```python
from build123d import *

# Parameters (mm, degrees)
SKETCH2_R               = 1.4
BOSS_EXTRUDE1_DEPTH     = 1.5
SKETCH5_R               = 1.6
CUT_EXTRUDE1_DEPTH      = 0.5
SKETCH3_R               = 1.4
SKETCH3_W               = 32.6
SKETCH3_H               = 52.5
BOSS_EXTRUDE2_DEPTH     = 1.5
SKETCH4_R               = 1.4
BOSS_EXTRUDE3_DEPTH     = 13.5
CHAMFER1_SIZE           = 2
CUT_EXTRUDE2_DEPTH      = 1
CUT_EXTRUDE2_DEPTH_BACK = 2.5


with BuildPart() as part:
    # Sketch2 → Boss-Extrude1 (new body)
    with BuildSketch(Plane(origin=(0, 0, 0), x_dir=(1, 0, 0), z_dir=(0, 1, 0))):
        with BuildLine():
            Line((-1.5, -1.5), (-1.5, 4.9))
            Line((-1.5, 4.9), (-4, 7.4))
            Line((-4, 7.4), (-4.5, 7.4))
            ThreePointArc((-4.5, 7.4), (-8.6, 11.5), (-4.5, 15.6))
            Line((-4.5, 15.6), (-4, 15.6))
            Line((-4, 15.6), (-1.5, 18.1))
            Line((-1.5, 18.1), (-1.5, 35.4))
            Line((-1.5, 35.4), (-4, 37.9))
            Line((-4, 37.9), (-4.5, 37.9))
            ThreePointArc((-4.5, 37.9), (-8.6, 42), (-4.5, 46.1))
            Line((-4.5, 46.1), (-4, 46.1))
            Line((-4, 46.1), (-1.5, 48.6))
            Line((-1.5, 48.6), (-1.5, 53.5))
            Line((-1.5, 53.5), (33.6, 53.5))
            Line((33.6, 53.5), (33.6, 48.6))
            Line((33.6, 48.6), (36.1, 46.1))
            Line((36.1, 46.1), (36.6, 46.1))
            ThreePointArc((36.6, 46.1), (40.7, 42), (36.6, 37.9))
            Line((36.6, 37.9), (36.1, 37.9))
            Line((36.1, 37.9), (33.6, 35.4))
            Line((33.6, 35.4), (33.6, 18.1))
            Line((33.6, 18.1), (36.1, 15.6))
            Line((36.1, 15.6), (36.6, 15.6))
            ThreePointArc((36.6, 15.6), (40.7, 11.5), (36.6, 7.4))
            Line((36.6, 7.4), (36.1, 7.4))
            Line((36.1, 7.4), (33.6, 4.9))
            Line((33.6, 4.9), (33.6, -1.5))
            Line((33.6, -1.5), (-1.5, -1.5))
        make_face()
        with Locations((-4.5, 42)):
            Circle(SKETCH2_R, mode=Mode.SUBTRACT)
        with Locations((-4.5, 11.5)):
            Circle(SKETCH2_R, mode=Mode.SUBTRACT)
        with Locations((36.6, 11.5)):
            Circle(SKETCH2_R, mode=Mode.SUBTRACT)
        with Locations((36.6, 42)):
            Circle(SKETCH2_R, mode=Mode.SUBTRACT)
    extrude(amount=-BOSS_EXTRUDE1_DEPTH)

    # Sketch5 → Cut-Extrude1 (cut)
    with BuildSketch(Plane(origin=(0, 0, 0), x_dir=(1, 0, 0), z_dir=(0, 1, 0))):
        with Locations((2.5, 42)):
            Circle(SKETCH5_R)
        with Locations((29.6, 42)):
            Circle(SKETCH5_R)
        with Locations((29.6, 11.5)):
            Circle(SKETCH5_R)
        with Locations((2.5, 11.5)):
            Circle(SKETCH5_R)
        Polygon((14.55, 36), (17.55, 36), (17.55, 39), (19.05, 39), (16.05, 42), (13.05, 39), (14.55, 39), align=None)
    extrude(amount=-CUT_EXTRUDE1_DEPTH, mode=Mode.SUBTRACT)

    # Sketch3 → Boss-Extrude2 (add)
    with BuildSketch(Plane(origin=(0, 0, 0), x_dir=(1, 0, 0), z_dir=(0, 1, 0))):
        with BuildLine():
            Line((-1.5, 53.5), (33.6, 53.5))
            Line((33.6, 53.5), (33.6, 48.6))
            Line((33.6, 48.6), (36.1, 46.1))
            Line((36.1, 46.1), (36.6, 46.1))
            ThreePointArc((36.6, 46.1), (40.7, 42), (36.6, 37.9))
            Line((36.6, 37.9), (36.1, 37.9))
            Line((36.1, 37.9), (33.6, 35.4))
            Line((33.6, 35.4), (33.6, 18.1))
            Line((33.6, 18.1), (36.1, 15.6))
            Line((36.1, 15.6), (36.6, 15.6))
            ThreePointArc((36.6, 15.6), (40.7, 11.5), (36.6, 7.4))
            Line((36.6, 7.4), (36.1, 7.4))
            Line((36.1, 7.4), (33.6, 4.9))
            Line((33.6, 4.9), (33.6, -1.5))
            Line((33.6, -1.5), (-1.5, -1.5))
            Line((-1.5, -1.5), (-1.5, 4.9))
            Line((-1.5, 4.9), (-4, 7.4))
            Line((-4, 7.4), (-4.5, 7.4))
            ThreePointArc((-4.5, 7.4), (-8.6, 11.5), (-4.5, 15.6))
            Line((-4.5, 15.6), (-4, 15.6))
            Line((-4, 15.6), (-1.5, 18.1))
            Line((-1.5, 18.1), (-1.5, 35.4))
            Line((-1.5, 35.4), (-4, 37.9))
            Line((-4, 37.9), (-4.5, 37.9))
            ThreePointArc((-4.5, 37.9), (-8.6, 42), (-4.5, 46.1))
            Line((-4.5, 46.1), (-4, 46.1))
            Line((-4, 46.1), (-1.5, 48.6))
            Line((-1.5, 48.6), (-1.5, 53.5))
        make_face()
        with Locations((-4.5, 42)):
            Circle(SKETCH3_R, mode=Mode.SUBTRACT)
        with Locations((36.6, 42)):
            Circle(SKETCH3_R, mode=Mode.SUBTRACT)
        with Locations((36.6, 11.5)):
            Circle(SKETCH3_R, mode=Mode.SUBTRACT)
        with Locations((-4.5, 11.5)):
            Circle(SKETCH3_R, mode=Mode.SUBTRACT)
        with Locations((16.05, 26)):
            Rectangle(SKETCH3_W, SKETCH3_H, mode=Mode.SUBTRACT)
    extrude(amount=BOSS_EXTRUDE2_DEPTH)

    # Sketch4 → Boss-Extrude3 (add)
    with BuildSketch(Plane(origin=(0, 1.5, 0), x_dir=(1, 0, 0), z_dir=(0, 1, 0))):
        with BuildLine():
            Line((-4.5, 46.1), (-0.25, 46.1))
            Line((-0.25, 46.1), (-0.25, 37.9))
            Line((-0.25, 37.9), (-4.5, 37.9))
            ThreePointArc((-4.5, 37.9), (-8.6, 42), (-4.5, 46.1))
        make_face()
        with Locations((-4.5, 42)):
            Circle(SKETCH4_R, mode=Mode.SUBTRACT)
        with BuildLine():
            Line((-4.5, 7.4), (-0.25, 7.4))
            Line((-0.25, 7.4), (-0.25, 15.6))
            Line((-0.25, 15.6), (-4.5, 15.6))
            ThreePointArc((-4.5, 15.6), (-8.6, 11.5), (-4.5, 7.4))
        make_face()
        with Locations((-4.5, 11.5)):
            Circle(SKETCH4_R, mode=Mode.SUBTRACT)
        with BuildLine():
            Line((32.35, 15.6), (32.35, 7.4))
            Line((32.35, 7.4), (36.6, 7.4))
            ThreePointArc((36.6, 7.4), (40.7, 11.5), (36.6, 15.6))
            Line((36.6, 15.6), (32.35, 15.6))
        make_face()
        with Locations((36.6, 11.5)):
            Circle(SKETCH4_R, mode=Mode.SUBTRACT)
        with BuildLine():
            Line((32.35, 46.1), (36.6, 46.1))
            ThreePointArc((36.6, 46.1), (40.7, 42), (36.6, 37.9))
            Line((36.6, 37.9), (32.35, 37.9))
            Line((32.35, 37.9), (32.35, 46.1))
        make_face()
        with Locations((36.6, 42)):
            Circle(SKETCH4_R, mode=Mode.SUBTRACT)
    extrude(amount=BOSS_EXTRUDE3_DEPTH)

    # Chamfer1
    chamfer1_edges = [part.edges().sort_by_distance(p)[0] for p in [
        (34.225, 1.5, -37.9),
        (34.225, 1.5, -46.1),
        (34.225, 1.5, -15.6),
        (34.225, 1.5, -7.4),
        (-2.125, 1.5, -7.4),
        (-2.125, 1.5, -15.6),
        (-2.125, 1.5, -37.9),
        (-2.125, 1.5, -46.1),
    ]]
    chamfer(chamfer1_edges, length=CHAMFER1_SIZE)

    # Sketch6 → Cut-Extrude2 (cut, two sides)
    with BuildSketch(Plane.XZ.offset(1.5)) as cut_extrude2_sk:
        Polygon((-1.266838493, -42), (-2.883419246, -39.2), (-6.116580754, -39.2), (-7.733161507, -42), (-6.116580754, -44.8), (-2.883419246, -44.8), align=None)
        Polygon((33.366838493, -42), (34.983419246, -44.8), (38.216580754, -44.8), (39.833161507, -42), (38.216580754, -39.2), (34.983419246, -39.2), align=None)
        Polygon((-1.266838493, -11.5), (-2.883419246, -8.7), (-6.116580754, -8.7), (-7.733161507, -11.5), (-6.116580754, -14.3), (-2.883419246, -14.3), align=None)
        Polygon((33.366838493, -11.5), (34.983419246, -14.3), (38.216580754, -14.3), (39.833161507, -11.5), (38.216580754, -8.7), (34.983419246, -8.7), align=None)
    extrude(amount=CUT_EXTRUDE2_DEPTH, mode=Mode.SUBTRACT)
    extrude(cut_extrude2_sk.sketch, amount=-CUT_EXTRUDE2_DEPTH_BACK, mode=Mode.SUBTRACT)


solid = part.part
```
Input: part model. Units: mm. Frame: model coordinates. A direction names the side the tool comes from. Round coordinates to 2 decimals unless told otherwise and drop trailing zeros. Loops run counter-clockwise (first coordinate to the right, second up) from the corner with the lowest first, then second, coordinate; pieces in that order, holes last. Notation, with made-up numbers: (55, -10) -> (68, -10) arc R23 ccw to (68, 3) -> close; hole circle Ø5 at (30.25, 66.5). An arc over 180 degrees is marked (long way). Use one line per item in the form item = value. Start each with the question number.
Item 1: Mould query, pull axis Z, two halves, no side actions, for faces 1 (the face through (39.014, -0.268, -43.42)), 2 (the face through (-2, 8, -46.1)), 3 (the face through (-1.5, 0, -51)), 4 (the face through (34.164, -0.268, -12.88)). Classes: pulls with the +Z half, pulls with the -Z half, needs draft (parallel to the pull), parting line crosses it, or undercut.
Item 2: Section query B-B on x = 2.5. Return the cut outline in (y, z), then the cut area to 4 significant figures.
Item 3: Section query A-A on y = 4.25. Return the cut outline in (x, z).
Item 4: Section query D-D on z = -16.5. Return the cut outline in (x, y).
Item 5: Material intervals for L1, parallel to X at y = -0.1, z = -11.5; L2, parallel to X at y = 8.75, z = -11.5; L3, parallel to Z at x = -4.5, y = 9, sorted ascending. Write a range as from..to.
Item 6: Contact query for flat-ended pins moving along their axis: pin 1 Ø3 at (x, y) = (-4.5, -0.5) entering from -Z; pin 2 Ø4.5 at (x, y) = (34, 5) entering from -Z; pin 3 Ø5 at (x, y) = (30, 12) entering from -Z; pin 4 Ø1 at (y, z) = (5, -35.5) entering from +X. Output: stop coordinate, or through.
Item 7: Section query C-C on z = -26. Return the cut outline in (x, y), then the cut area to 3 significant figures.
Item 8: Set-up query: faces 5 (the face through (34.164, -0.268, -43.38)), 6 (the face through (-1.7, 2.7, -37.1)), 7 (the face through (28, -0.25, -42.07)). Return all of +Z, -Z, +X, -X, +Y, -Y with unobstructed straight access to the full face (end or side cutting, diameter ignored); none if empty.
Ans:
q1.face_1 = undercut
q1.face_2 = pulls with the -Z half
q1.face_3 = needs draft
q1.face_4 = undercut
q2.outline = (-1.5, -53.5) -> (1.5, -53.5) -> (1.5, -52.25) -> (0, -52.25) -> (0, -43.6) -> (-0.5, -43.6) -> (-0.5, -40.4) -> (0, -40.4) -> (0, -13.1) -> (-0.5, -13.1) -> (-0.5, -9.9) -> (0, -9.9) -> (0, 0.25) -> (1.5, 0.25) -> (1.5, 1.5) -> (-1.5, 1.5) -> close
q2.area = 83.05 mm^2
q3.outline = (-4.5, -46.1) -> (-0.25, -46.1) -> (-0.25, -37.9) -> (-4.5, -37.9) arc R4.1 ccw to start; (-4.5, -15.6) -> (-0.25, -15.6) -> (-0.25, -7.4) -> (-4.5, -7.4) arc R4.1 ccw to start; (32.35, -46.1) -> (36.6, -46.1) arc R4.1 ccw to (36.6, -37.9) -> (32.35, -37.9) -> close; (32.35, -15.6) -> (36.6, -15.6) arc R4.1 ccw to (36.6, -7.4) -> (32.35, -7.4) -> close; hole circle Ø2.8 at (-4.5, -42); hole circle Ø2.8 at (-4.5, -11.5); hole circle Ø2.8 at (36.6, -42); hole circle Ø2.8 at (36.6, -11.5)
q4.outline = (-3.1, -1.5) -> (35.2, -1.5) -> (35.2, 2.6) -> (32.35, 2.6) -> (32.35, 0) -> (-0.25, 0) -> (-0.25, 2.6) -> (-3.1, 2.6) -> close
q5.L1 = -8.6..-7.73, -1.27..0.9, 4.1..28, 31.2..33.37, 39.83..40.7
q5.L2 = -8.6..-5.9, -3.1..-0.25, 32.35..35.2, 38..40.7
q5.L3 = -46.1..-43.4, -40.6..-37.9, -15.6..-12.9, -10.1..-7.4
q6.pin_1 = -47.1
q6.pin_2 = -46.85
q6.pin_3 = -46.1
q6.pin_4 = through
q7.outline = (-1.5, -1.5) -> (33.6, -1.5) -> (33.6, 1.5) -> (32.35, 1.5) -> (32.35, 0) -> (-0.25, 0) -> (-0.25, 1.5) -> (-1.5, 1.5) -> close
q7.area = 56.4 mm^2
q8.face_5 = -Y
q8.face_6 = +X, -X, +Y
q8.face_7 = +Y
